```python
from build123d import *

# Parameters (mm, degrees)
F0_W     = 20
F0_H     = 20
F1_DEPTH = 500
F2_W     = 2.6593398282
F2_H     = 5.68
F2_W_2   = 2.84
F2_H_2   = 2.6593398282
F2_W_3   = 1.64
F2_H_3   = 1.64
F2_H_4   = 1.8
F3_DEPTH = 1000
F5_DEPTH = 100
F6_R     = 1


with BuildPart() as f1:
    # F0 (on Front) → F1 (new body)
    with BuildSketch(Plane.XZ):
        with Locations((10, 10)):
            Rectangle(F0_W, F0_H)
    extrude(amount=F1_DEPTH)

    # F2 (on face) → F3 (cut)
    with BuildSketch(Plane.XZ.offset(500)):
        with BuildLine():
            ThreePointArc((11.9173232366, 9.1433369352), (12.0538231176, 9.5620381277), (12.1, 10))
            ThreePointArc((12.1, 10), (12.0538231176, 10.4379618723), (11.9173232366, 10.8566630648))
            Line((11.9173232366, 10.8566630648), (11.0606601718, 10))
            Line((11.0606601718, 10), (11.9173232366, 9.1433369352))
        make_face()
        with BuildLine():
            Line((11.0606601718, 10), (11.9173232366, 10.8566630648))
            ThreePointArc((11.9173232366, 10.8566630648), (11.4849242405, 11.4849242405), (10.8566630648, 11.9173232366))
            Line((10.8566630648, 11.9173232366), (10, 11.0606601718))
            Line((10, 11.0606601718), (11.0606601718, 10))
        make_face()
        with BuildLine():
            ThreePointArc((11.4849242405, 8.5150757595), (11.7298843892, 8.80941191), (11.9173232366, 9.1433369352))
            Line((11.9173232366, 9.1433369352), (11.0606601718, 10))
            Line((11.0606601718, 10), (10.5303300859, 9.4696699141))
            Line((10.5303300859, 9.4696699141), (11.4849242405, 8.5150757595))
        make_face()
        with BuildLine():
            Line((10, 11.0606601718), (10.8566630648, 11.9173232366))
            ThreePointArc((10.8566630648, 11.9173232366), (10.4379618723, 12.0538231176), (10, 12.1))
            Line((10, 12.1), (10, 11.0606601718))
        make_face()
        Polygon((16.56, 15.4993398282), (13.9006601718, 12.84), (16.56, 12.84), align=None)
        with Locations((15.2303300859, 10)):
            Rectangle(F2_W, F2_H)
        Polygon((10.5303300859, 9.4696699141), (11.0606601718, 10), (10, 11.0606601718), (10, 10), align=None)
        with BuildLine():
            ThreePointArc((10.8566630648, 8.0826767634), (11.19058809, 8.2701156108), (11.4849242405, 8.5150757595))
            Line((11.4849242405, 8.5150757595), (10.5303300859, 9.4696699141))
            Line((10.5303300859, 9.4696699141), (10, 8.9393398282))
            Line((10, 8.9393398282), (10.8566630648, 8.0826767634))
        make_face()
        Polygon((16.56, 7.16), (13.9006601718, 7.16), (16.56, 4.5006601718), align=None)
        with BuildLine():
            Line((10, 11.0606601718), (10, 12.1))
            ThreePointArc((10, 12.1), (9.5620381277, 12.0538231176), (9.1433369352, 11.9173232366))
            Line((9.1433369352, 11.9173232366), (10, 11.0606601718))
        make_face()
        with BuildLine():
            Line((9.4696699141, 10.5303300859), (10, 11.0606601718))
            Line((10, 11.0606601718), (9.1433369352, 11.9173232366))
            ThreePointArc((9.1433369352, 11.9173232366), (8.80941191, 11.7298843892), (8.5150757595, 11.4849242405))
            Line((8.5150757595, 11.4849242405), (9.4696699141, 10.5303300859))
        make_face()
        Polygon((10, 10), (10, 11.0606601718), (9.4696699141, 10.5303300859), align=None)
        Polygon((12.84, 16.56), (12.84, 13.9006601718), (15.4993398282, 16.56), align=None)
        with Locations((11.42, 15.2303300859)):
            Rectangle(F2_W_2, F2_H_2)
        with Locations((17.38, 14.1696699141)):
            Rectangle(F2_W_3, F2_H_2)
        with Locations((17.38, 10)):
            Rectangle(F2_W_3, F2_H)
        Polygon((10, 8.9393398282), (10.5303300859, 9.4696699141), (10, 10), align=None)
        with BuildLine():
            ThreePointArc((10, 7.9), (10.4379618723, 7.9461768824), (10.8566630648, 8.0826767634))
            Line((10.8566630648, 8.0826767634), (10, 8.9393398282))
            Line((10, 8.9393398282), (10, 7.9))
        make_face()
        with Locations((17.38, 5.8303300859)):
            Rectangle(F2_W_3, F2_H_2)
        with Locations((8.58, 15.2303300859)):
            Rectangle(F2_W_2, F2_H_2)
        Polygon((10, 10), (9.4696699141, 10.5303300859), (8.9393398282, 10), (10, 8.9393398282), align=None)
        with BuildLine():
            Line((8.9393398282, 10), (9.4696699141, 10.5303300859))
            Line((9.4696699141, 10.5303300859), (8.5150757595, 11.4849242405))
            ThreePointArc((8.5150757595, 11.4849242405), (8.2701156108, 11.19058809), (8.0826767634, 10.8566630648))
            Line((8.0826767634, 10.8566630648), (8.9393398282, 10))
        make_face()
        with Locations((14.1696699141, 17.38)):
            Rectangle(F2_W, F2_H_3)
        with Locations((11.42, 17.38)):
            Rectangle(F2_W_2, F2_H_3)
        Polygon((20, 12.84), (18.2, 12.84), (18.2, 7.16), (20, 7.16), (20, 10), align=None)
        Polygon((20, 14.64), (18.2, 12.84), (20, 12.84), align=None)
        with BuildLine():
            Line((9.1433369352, 8.0826767634), (10, 8.9393398282))
            Line((10, 8.9393398282), (8.9393398282, 10))
            Line((8.9393398282, 10), (8.0826767634, 9.1433369352))
            ThreePointArc((8.0826767634, 9.1433369352), (8.5150757595, 8.5150757595), (9.1433369352, 8.0826767634))
        make_face()
        with BuildLine():
            Line((10, 7.9), (10, 8.9393398282))
            Line((10, 8.9393398282), (9.1433369352, 8.0826767634))
            ThreePointArc((9.1433369352, 8.0826767634), (9.5620381277, 7.9461768824), (10, 7.9))
        make_face()
        Polygon((15.4993398282, 3.44), (12.84, 6.0993398282), (12.84, 3.44), align=None)
        with Locations((11.42, 4.7696699141)):
            Rectangle(F2_W_2, F2_H_2)
        Polygon((20, 7.16), (18.2, 7.16), (20, 5.36), align=None)
        Polygon((4.5006601718, 16.56), (7.16, 13.9006601718), (7.16, 16.56), align=None)
        with Locations((8.58, 17.38)):
            Rectangle(F2_W_2, F2_H_3)
        with BuildLine():
            Line((8.0826767634, 9.1433369352), (8.9393398282, 10))
            Line((8.9393398282, 10), (8.0826767634, 10.8566630648))
            ThreePointArc((8.0826767634, 10.8566630648), (7.9, 10), (8.0826767634, 9.1433369352))
        make_face()
        Polygon((12.84, 20), (12.84, 18.2), (14.64, 20), align=None)
        with Locations((11.42, 19.1)):
            Rectangle(F2_W_2, F2_H_4)
        with Locations((8.58, 4.7696699141)):
            Rectangle(F2_W_2, F2_H_2)
        with Locations((14.1696699141, 2.62)):
            Rectangle(F2_W, F2_H_3)
        with Locations((11.42, 2.62)):
            Rectangle(F2_W_2, F2_H_3)
        with Locations((5.8303300859, 17.38)):
            Rectangle(F2_W, F2_H_3)
        with Locations((8.58, 19.1)):
            Rectangle(F2_W_2, F2_H_4)
        Polygon((7.16, 3.44), (7.16, 6.0993398282), (4.5006601718, 3.44), align=None)
        with Locations((8.58, 2.62)):
            Rectangle(F2_W_2, F2_H_3)
        with Locations((11.42, 0.9)):
            Rectangle(F2_W_2, F2_H_4)
        Polygon((14.64, 0), (12.84, 1.8), (12.84, 0), align=None)
        Polygon((3.44, 12.84), (6.0993398282, 12.84), (3.44, 15.4993398282), align=None)
        with Locations((4.7696699141, 10)):
            Rectangle(F2_W, F2_H)
        Polygon((5.36, 20), (7.16, 18.2), (7.16, 20), align=None)
        Polygon((3.44, 4.5006601718), (6.0993398282, 7.16), (3.44, 7.16), align=None)
        with Locations((5.8303300859, 2.62)):
            Rectangle(F2_W, F2_H_3)
        with Locations((8.58, 0.9)):
            Rectangle(F2_W_2, F2_H_4)
        with Locations((2.62, 14.1696699141)):
            Rectangle(F2_W_3, F2_H_2)
        with Locations((2.62, 10)):
            Rectangle(F2_W_3, F2_H)
        with Locations((2.62, 5.8303300859)):
            Rectangle(F2_W_3, F2_H_2)
        Polygon((7.16, 0), (7.16, 1.8), (5.36, 0), align=None)
        Polygon((0, 12.84), (1.8, 12.84), (0, 14.64), align=None)
        Polygon((1.8, 7.16), (1.8, 12.84), (0, 12.84), (0, 10), (0, 7.16), align=None)
        Polygon((0, 5.36), (1.8, 7.16), (0, 7.16), align=None)
    extrude(amount=-F3_DEPTH, mode=Mode.SUBTRACT)

    # F4 (on face) → F5 (cut)
    with BuildSketch(Plane.XZ.offset(500)):
        Polygon((3.4306601718, 1.8), (1.8, 3.4306601718), (1.8, 1.8), align=None)
        Polygon((1.8, 18.2), (1.8, 16.5693398282), (3.4306601718, 18.2), align=None)
        Polygon((18.2, 18.2), (16.5693398282, 18.2), (18.2, 16.5693398282), align=None)
        Polygon((18.2, 3.4306601718), (16.5693398282, 1.8), (18.2, 1.8), align=None)
    extrude(amount=-F5_DEPTH, mode=Mode.SUBTRACT)

    # F6
    f6_edges = [f1.edges().sort_by_distance(p)[0] for p in [
        (20, -250, 20),
        (20, -250, 0),
        (0, -250, 20),
        (0, -250, 0),
    ]]
    fillet(f6_edges, radius=F6_R)


solid = f1.part
```
Geometry check sheet. Reference: the model listing, model coordinates, mm. Give positions to 0.01 mm unless a question says otherwise; leave off trailing zeros.
1. Section check A-A, the plane y = -406.5. Give the number of separate pieces and of enclosed holes in the cut face, and give its area (3 significant figures).
2. Gauge pin test, flat ends, axial feed: pin 1 Ø8 at (y, z) = (-413.5, 10.5) entering from -X; pin 2 Ø2 at (x, y) = (14, -191.5) entering from +Z; pin 3 Ø6 at (x, y) = (10.5, -205.5) entering from +Z; pin 4 Ø4.5 at (y, z) = (-266.5, 9) entering from +X. Record the tip position at first contact, or that the pin passes through.
3. Thickness scan on L1, parallel to X at y = -360.5, z = 9.5; L2, parallel to Z at x = 9, y = -114.5; L3, parallel to X at y = -284, z = 3. Record the ranges inside material, lowest first.
Values follow:
1. separate pieces: 1
1. enclosed holes: 5
1. area: 165 mm2
2. pin 1: stops at x = 0.14
2. pin 2: stops at z = 20
2. pin 3: stops at z = 18.86
2. pin 4: stops at x = 18.61
3. L1: x = 6.1 to 7.96, 12.04 to 13.9
3. L2: z = 6.1 to 8.15, 11.85 to 13.9
3. L3: x = 0 to 4.5, 15.5 to 20
